For this review, take the finished solid that the model builds, in its own axes (mm). A direction names the side the tool comes from. Coordinates: 2 decimals unless noted, no trailing zeros. Order: outer loops, then holes, each group sorted by start corner. A loop starts at its lowest first (then second) coordinate and runs counter-clockwise, first axis right, second up. Notation, with made-up numbers: (-7, 76.5) -> (33, 76.5) arc R38 ccw to (33, 114.5) -> close; hole circle Ø9 at (82.25, 78). An arc over 180 degrees is marked (long way). Write item = value, one per line. Start each with the question number.
1) Machinability: for faces 1 (the face through (-0.69, -3.1, -11.52)), 2 (the face through (0, 3, -81.28)), which of the approach directions +Z, -Z, +X, -X, +Y, -Y give a long, thin tool a straight path to every point of the face, cutting with its end or side? Answer none if there is none.
2) Insertion check: pin 1 Ø1 at (y, z) = (0, -52) entering from +X. The pin has a flat end and moves straight along its axis. Give the tip position at first contact, or say it passes through.
3) Draft analysis for pull direction Z (two halves, no side actions). For faces 3 (the face through (0, 0, -95.25)), 4 (the face through (0, 0, 0)), 5 (the face through (-0.69, -3.1, -31.02)), 6 (the face through (0, 3, -38.1)), state which applies: +Z half, -Z half, draft (parallel to the pull), parting line (faces both ways), or undercut.
4) Wall thickness on probe 1 along Z at (x, y) = (1.25, -2.25); probe 2 along Y at (x, z) = (0.25, -37): over which ranges is each line inside the solid? List them lowest first. Write a range as [from, to].
5) Consider section C-C on z = -40.5. Give the boundary of the cut face in (x, y), and give its area (3 significant figures).
6) Consider section A-A on x = 0. Give the boundary of the cut face in (y, z) (3 decimals).
7) Consider section D-D on z = -19. Give the boundary of the cut face in (x, y) (3 decimals), and give its area (3 significant figures).
Autodesk Inventor part; units mm, degrees
ref_plane "YZ Plane" through (0, 0, 0) normal (1, 0, 0) x (0, 1, 0)
ref_plane "XY Plane" through (0, 0, 0) normal (0, 0, 1) x (1, 0, 0)
sketch "Sketch1" plane through (0, 0, 0) normal (0, 0, 1) x (1, 0, 0)
  circle A0 centre (0, 0) radius 3.175
  dimension "d0" = 6.35
extrude "Extrusion1" add sketch "Sketch1" against normal blind 95.25
ref_plane "Work Plane5" through (0, 0, -81.28) normal (0, 0, -1) x (-1, 0, 0)
sketch "Sketch6" plane through (0, 0, -81.28) normal (0, 0, -1) x (-1, 0, 0)
  circle A0 centre (0, 0) radius 2.54
  circle A1 centre (0, 0) radius 3.175
  dimension "d11" = 5.08
  dimension "d12" = 6.35
extrude "Extrusion4" cut sketch "Sketch6" against normal blind 43.18
ref_plane "Work Plane6" through (0, 0, -84.074) normal (0, 0, -1) x (-1, 0, 0)
sketch "Sketch7" plane through (0, 0, -84.074) normal (0, 0, -1) x (-1, 0, 0)
  circle A0 centre (0, 0) radius 3.175
  circle A1 centre (0, 0) radius 2.921
  dimension "d16" = 6.35
  dimension "d17" = 5.842
extrude "Extrusion5" cut sketch "Sketch7" against normal blind 0.762
ref_plane "Work Plane7" through (0, 0, -23.368) normal (0, 0, -1) x (-1, 0, 0)
sketch "Sketch8" plane through (0, 0, -23.368) normal (0, 0, -1) x (-1, 0, 0)
  circle A0 centre (0, 0) radius 3.175
  circle A1 centre (0, 0) radius 2.921
  dimension "d21" = 6.35
  dimension "d22" = 5.842
extrude "Extrusion6" cut sketch "Sketch8" along normal blind 0.762
properties part number "ShaftStraight" material "Aluminum-6061"
Answer sheet:
q1.face_1 = +Z, -Z
q1.face_2 = none
q2.pin_1 = 2.54
q3.face_3 = -Z half
q3.face_4 = +Z half
q3.face_5 = draft
q3.face_6 = undercut
q4.probe_1 = [-95.25, -81.28], [-38.1, 0]
q4.probe_2 = [-3.17, 3.17]
q5.outline = circle Ø5.08 at (0, 0)
q5.area = 20.3 mm2
q6.outline = (-3.175, -95.25) -> (3.175, -95.25) -> (3.175, -84.074) -> (2.921, -84.074) -> (2.921, -83.312) -> (3.175, -83.312) -> (3.175, -81.28) -> (2.54, -81.28) -> (2.54, -38.1) -> (3.175, -38.1) -> (3.175, -24.13) -> (2.921, -24.13) -> (2.921, -23.368) -> (3.175, -23.368) -> (3.175, 0) -> (-3.175, 0) -> (-3.175, -23.368) -> (-2.921, -23.368) -> (-2.921, -24.13) -> (-3.175, -24.13) -> (-3.175, -38.1) -> (-2.54, -38.1) -> (-2.54, -81.28) -> (-3.175, -81.28) -> (-3.175, -83.312) -> (-2.921, -83.312) -> (-2.921, -84.074) -> (-3.175, -84.074) -> close
q7.outline = circle Ø6.35 at (0, 0)
q7.area = 31.7 mm2
